Input: dimensioned drawing with shaded views. Units: mm. Origin: part minimum x, y, z. Coordinates: 2 decimals unless noted, no trailing zeros. Loops run counter-clockwise (first coordinate to the right, second up) from the corner with the lowest first, then second, coordinate; pieces in that order, holes last.
Item 1: Pull-direction query (X, two-part tool) for the marked faces 1, 2, 3 and 4; classes: released by +X, released by -X, zero draft, split by the parting line, or undercut.
Item 2: Section A-A on z = 3.7. Return loops of the section in (x, y), and give its area (3 significant figures).
Item 3: Section B-B on x = 14. Return loops of the section in (y, z), and give its area (3 significant figures).
Item 4: Section C-C on y = 13. Return loops of the section in (x, z).
Item 5: Ray query, line 1 along Z through (x, y) = (4, 4.5); line 2 along Y through (x, z) = (14, 3.65); line 3 along X through (y, z) = (11.5, 3.05). Return the intervals inside material, ascending.
Item 6: Section D-D on y = 22.5. Return loops of the section in (x, z), and give its area (3 significant figures).
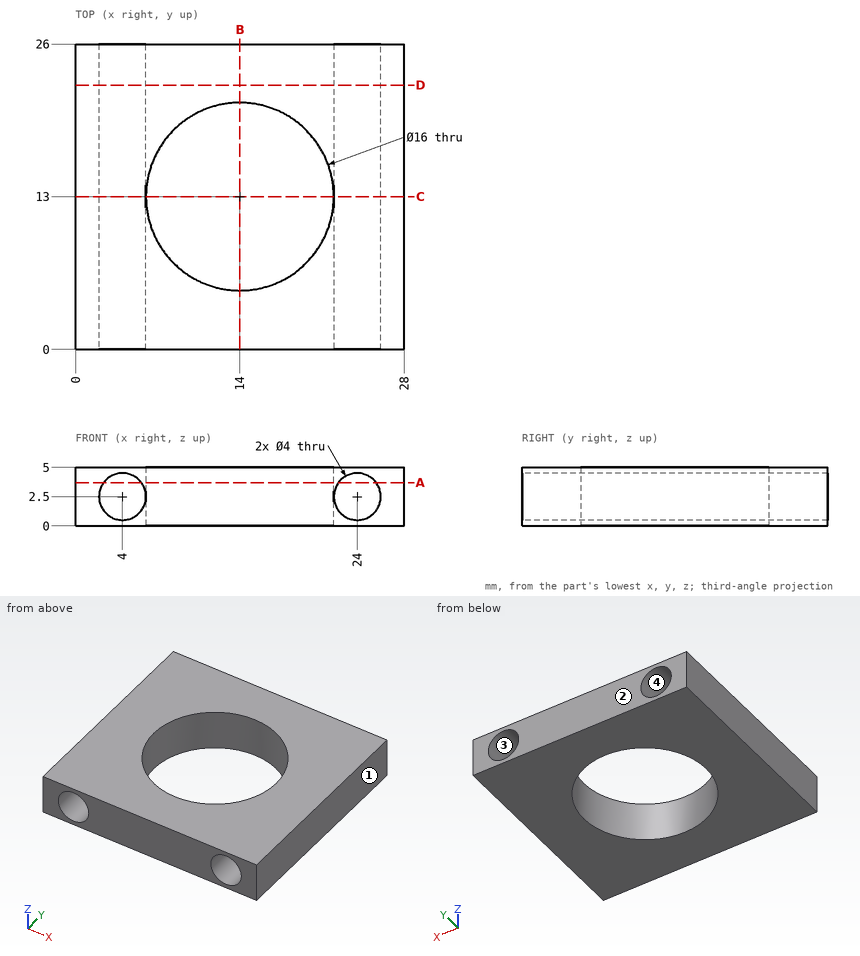
Results found:
1. face 1: released by +X
1. face 2: zero draft
1. face 3: undercut
1. face 4: undercut
2. outline: (0, 0) - (2.4, 0) - (2.4, 26) - (0, 26) - close; (5.6, 0) - (22.4, 0) - (22.4, 26) - (5.6, 26) - close; (25.6, 0) - (28, 0) - (28, 26) - (25.6, 26) - close; hole circle Ø16 at (14, 13)
2. area: 361 mm2
3. outline: (0, 0) - (5, 0) - (5, 5) - (0, 5) - close; (21, 0) - (26, 0) - (26, 5) - (21, 5) - close
3. area: 50.0 mm2
4. outline: (0, 0) - (6, 0) - (6, 5) - (0, 5) - close; (22, 0) - (28, 0) - (28, 5) - (22, 5) - close; hole circle Ø4 at (4, 2.5); hole circle Ø4 at (24, 2.5)
5. line 1: z = 0 to 0.5, 4.5 to 5
5. line 2: y = 0 to 5, 21 to 26
5. line 3: x = 0 to 2.08, 5.92 to 6.14, 21.86 to 22.08, 25.92 to 28
6. outline: (0, 0) - (28, 0) - (28, 5) - (0, 5) - close; hole circle Ø4 at (4, 2.5); hole circle Ø4 at (24, 2.5)
6. area: 115 mm2
